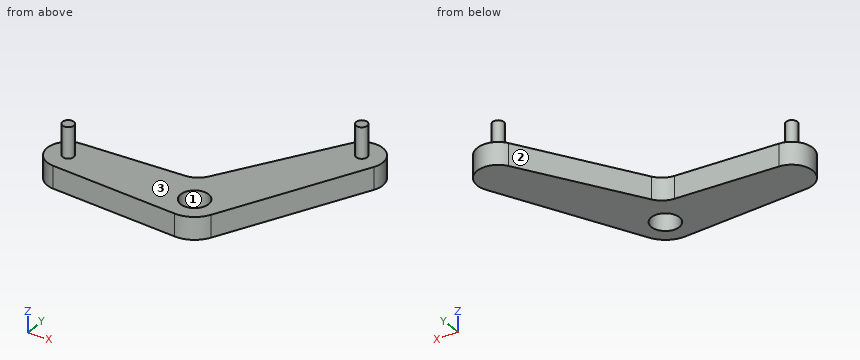
from build123d import *

# Parameters (mm, degrees)
EXTRUDE_1_DEPTH     = 16
SKETCH_2_R          = 4
EXTRUDE_2_DEPTH     = 22
SKETCH_3_R          = 10
CUT_EXTRUDE_1_DEPTH = 16


with BuildPart() as part:
    # 草图1 → 凸台-拉伸1 (new body)
    with BuildSketch(Plane.XY):
        with BuildLine():
            Line((68.765313927, 89.135523785), (17.753751903, -9.208924659))
            ThreePointArc((17.753751903, -9.208924659), (9.909075677, -17.372686011), (-1.111111111, -19.969111951))
            Line((-1.111111111, -19.969111951), (-90.833333333, -14.976833963))
            ThreePointArc((-90.833333333, -14.976833963), (-105, 0), (-90.833333333, 14.976833963))
            Line((-90.833333333, 14.976833963), (-19.005850553, 18.973422013))
            ThreePointArc((-19.005850553, 18.973422013), (-12.271196702, 20.999365274), (-7.200154901, 25.872202603))
            Line((-7.200154901, 25.872202603), (42.810971014, 104.120270653))
            ThreePointArc((42.810971014, 104.120270653), (62.95, 109.032598336), (68.765313927, 89.135523785))
        make_face()
    extrude(amount=EXTRUDE_1_DEPTH)

    # 草图2 → 凸台-拉伸2 (add)
    with BuildSketch(Plane.XY.offset(16)):
        with Locations(Location((-90, 0, 0), (0, 0, 180))):
            Circle(SKETCH_2_R)
        with Locations(Location((55.45, 96.04221728, 0), (0, 0, 180))):
            Circle(SKETCH_2_R)
    extrude(amount=EXTRUDE_2_DEPTH)

    # 草图3 → 切除-拉伸1 (cut)
    with BuildSketch(Plane.XY):
        Circle(SKETCH_3_R)
    extrude(amount=CUT_EXTRUDE_1_DEPTH, mode=Mode.SUBTRACT)


solid = part.part
Check sheet for the modelled part. Datum: model origin and axes. Units: mm. Face numbers are marked on the shaded views. Coordinates: 2 decimals unless noted, no trailing zeros. Write each loop counter-clockwise with the first axis right and the second up, starting at its lowest first coordinate (ties: lowest second). Pieces come first, ordered by that corner, then holes. Notation, with made-up numbers: M 80.5,48 L 113.5,48 A15 ccw 113.5,66 Z; hole C 22.5,81.5 d1. An arc over 180 degrees is marked long. Answer as CSV lines item,"result".
Q1. Go/stop test with flat-tipped pins: pin 1 (4 mm diameter, centred on y = 14.5, z = 10.5, fed in from -X); pin 2 (3 mm diameter, centred on y = 94, z = 19, fed in from +X); pin 3 (2 mm diameter, centred on x = -20.5, y = 17, fed in from +Z); pin 4 (4 mm diameter, centred on x = 7, y = 31, fed in from -Z). Record where each tip stops, or that it passes through.
Check result:
pin 1,"x = -98.29"
pin 2,"x = 59.41"
pin 3,"z = 16"
pin 4,"z = 0"
Q2. Cross-section at A-A (z = 9). Record the boundary of the cut face in (x, y), then the cut area to 3 significant figures.
Check result:
outline,"M -90.83,-14.98 L -1.11,-19.97 A20 ccw 17.75,-9.21 L 68.77,89.14 A15 ccw 42.81,104.12 L -7.2,25.87 A15 cw -19.01,18.97 L -90.83,14.98 A15 ccw Z; hole C 0,0 d20"
area,"7,430 mm^2"
Q3. Material ranges on probe 1 along Z at (x, y) = (-80, 7); probe 2 along Y at (x, z) = (0, 5.5); probe 3 along Y at (x, z) = (-97.5, 13.5), recorded low to high. Write a range as from..to.
Check result:
probe 1,"0..16"
probe 2,"-20..-10, 10..37.14"
probe 3,"-12.99..12.99"
Q4. Cross-section at B-B (y = 0). Record the boundary of the cut face in (x, z), then the cut area to 3 significant figures.
Check result:
outline,"M -105,0 L -10,0 L -10,16 L -86,16 L -86,38 L -94,38 L -94,16 L -105,16 Z; M 10,0 L 22.53,0 L 22.53,16 L 10,16 Z"
area,"1,900 mm^2"
Q5. Cross-section at C-C (x = 7.5). Record the boundary of the cut face in (y, z), then the cut area to 3 significant figures.
Check result:
outline,"M -18.54,0 L -6.61,0 L -6.61,16 L -18.54,16 Z; M 6.61,0 L 48.87,0 L 48.87,16 L 6.61,16 Z"
area,"867 mm^2"
Q6. Mould release check, pull along Y, two halves, no side actions. Record for the marked faces 1, 2 and 3: released by +Y, released by -Y, zero draft, split by the parting line, or undercut.
Check result:
face 1,"undercut"
face 2,"released by +Y"
face 3,"zero draft"
Q7. Cross-section at D-D (x = 55.45). Record the boundary of the cut face in (y, z), then the cut area to 3 significant figures.
Check result:
outline,"M 63.47,0 L 111.04,0 L 111.04,16 L 100.04,16 L 100.04,38 L 92.04,38 L 92.04,16 L 63.47,16 Z"
area,"937 mm^2"
